from build123d import *

# Parameters (mm, degrees)
F0_W     = 25
F0_H     = 35
F1_DEPTH = 5
F2_W     = 25
F2_H     = 35
F3_DEPTH = 10
F4_R     = 5
F5_T     = 2.5


# Not quite as in the source:
# - a shell that OpenCascade refuses in one call is made with other operations: the cavity is built on its own and cut out


with BuildPart() as f1:
    # F0 (on Top) → F1 (new body)
    with BuildSketch(Plane.XY):
        Rectangle(F0_W, F0_H)
    extrude(amount=F1_DEPTH)

    # F2 (on Top) → F3 (join)
    with BuildSketch(Plane.XY):
        Rectangle(F2_W, F2_H)
    extrude(amount=F3_DEPTH)

    # F4
    f4_edges = [f1.edges().sort_by_distance(p)[0] for p in [
        (-12.5, 0, 10),
        (12.5, 0, 10),
    ]]
    fillet(f4_edges, radius=F4_R)

    # F5: shell of thickness 2.5, made by hand


with BuildPart() as f5_core1:
    # F5_t2: copy of F1
    add(f1.part)

    # the walls: a layer under each face that stays
    f5_faces = [f5_core1.faces().sort_by_distance(p)[0] for p in [
        (0, -17.5, 5),
        (-12.5, 0, 2.5),
        (0, 0, 0),
        (0, 0, 10),
        (12.5, 0, 2.5),
        (0, 17.5, 5),
    ]]
    thicken(f5_faces, amount=-F5_T, mode=Mode.SUBTRACT)


with BuildPart() as f1_1:
    add(f1.part)

    # what is left inside the walls is the cavity
    f5_cavity = [f5_core1.part.solids().sort_by_distance(p)[0] for p in [
        (0, -5, 2.525),
    ]]
    add(f5_cavity, mode=Mode.SUBTRACT)


solid = f1_1.part
CAD build for the part. Positions are in the model's coordinates, mm. A direction names the side the tool comes from. Round coordinates to 2 decimals unless told otherwise and drop trailing zeros. Order: outer loops, then holes, each group sorted by start corner. A loop starts at its lowest first (then second) coordinate and runs counter-clockwise, first axis right, second up. Notation, with made-up numbers: (-26.75, 3) -> (2.25, 3) arc R13 ccw to (2.25, 8) -> close; hole circle Ø3 at (81, 3.5). An arc over 180 degrees is marked (long way). Write item = value, one per line. Start each with the question number.
(1) Pull direction Z, two halves, no side cores. Call faces 4 (the flat face through (0, 0, 7.5)), 5 (the flat face through (0, -17.5, 5)), 6 (the flat face through (0, 0, 0)): released by +Z, released by -Z, zero draft, split by the parting line, or undercut.
(2) Cut at B-B, the plane x = 1.25. List the corners of the cut face in (y, z).
(3) Which spindle directions (+Z, -Z, +X, -X, +Y, -Y) get a long thin tool onto all of the face, cutting with end or side? Do faces 1 (the flat face through (11, 0, 5)), 2 (the flat face through (10, 0, 4)), 3 (the flat face through (0, 0, 2.5)). Say none if no direction does.
(4) Pin check, flat tips, straight feed: P1, Ø3, axis at y = -5.5, z = 8.5, coming from the +X side; P2, Ø2, axis at x = 11.5, y = -3.5, coming from the +Z side; P3, Ø0.8, axis at y = -3, z = 9.5, coming from the -X side; P4, Ø4.5, axis at x = 3.5, y = -2, coming from the -Z side. Stop position of each tip, or through.
(5) Probe line 1 (Y direction, x = -1.25, z = 6); line 2 (Z direction, x = -2.5, y = 10); line 3 (X direction, y = -10, z = 4.75). List the from-to ranges inside material, lowest first. Write a range as [from, to].
(6) Cut at C-C, the plane y = -7.5. List the corners of the cut face in (x, z).
(7) Cut at A-A, the plane z = 3.75. List the corners of the cut face in (x, y).
(8) Cut at D-D, the plane x = -9. List the corners of the cut face in (y, z), then the cut area to 3 significant figures.
Model answer:
q1.face_4 = undercut
q1.face_5 = zero draft
q1.face_6 = released by -Z
q2.outline = (-17.5, 0) -> (17.5, 0) -> (17.5, 10) -> (-17.5, 10) -> close; hole (-15, 2.5) -> (15, 2.5) -> (15, 7.5) -> (-15, 7.5) -> close
q3.face_1 = +Z, +X, -X
q3.face_2 = +Z
q3.face_3 = none
q4.P1 = 7.5
q4.P2 = 5
q4.P3 = -7.5
q4.P4 = 0
q5.line_1 = [-17.5, -15], [15, 17.5]
q5.line_2 = [0, 2.5], [7.5, 10]
q5.line_3 = [-12.5, -10], [10, 12.5]
q6.outline = (-12.5, 0) -> (12.5, 0) -> (12.5, 5) -> (10, 5) -> (10, 2.5) -> (-10, 2.5) -> (-10, 5) -> (-12.5, 5) -> close; (-7.5, 7.5) -> (7.5, 7.5) -> (7.5, 10) -> (-7.5, 10) -> close
q7.outline = (-12.5, -17.5) -> (12.5, -17.5) -> (12.5, 17.5) -> (-12.5, 17.5) -> close; hole (-10, -15) -> (10, -15) -> (10, 15) -> (-10, 15) -> close
q8.outline = (-17.5, 0) -> (17.5, 0) -> (17.5, 9.77) -> (15, 9.77) -> (15, 2.5) -> (-15, 2.5) -> (-15, 9.77) -> (-17.5, 9.77) -> close
q8.area = 124 mm2
